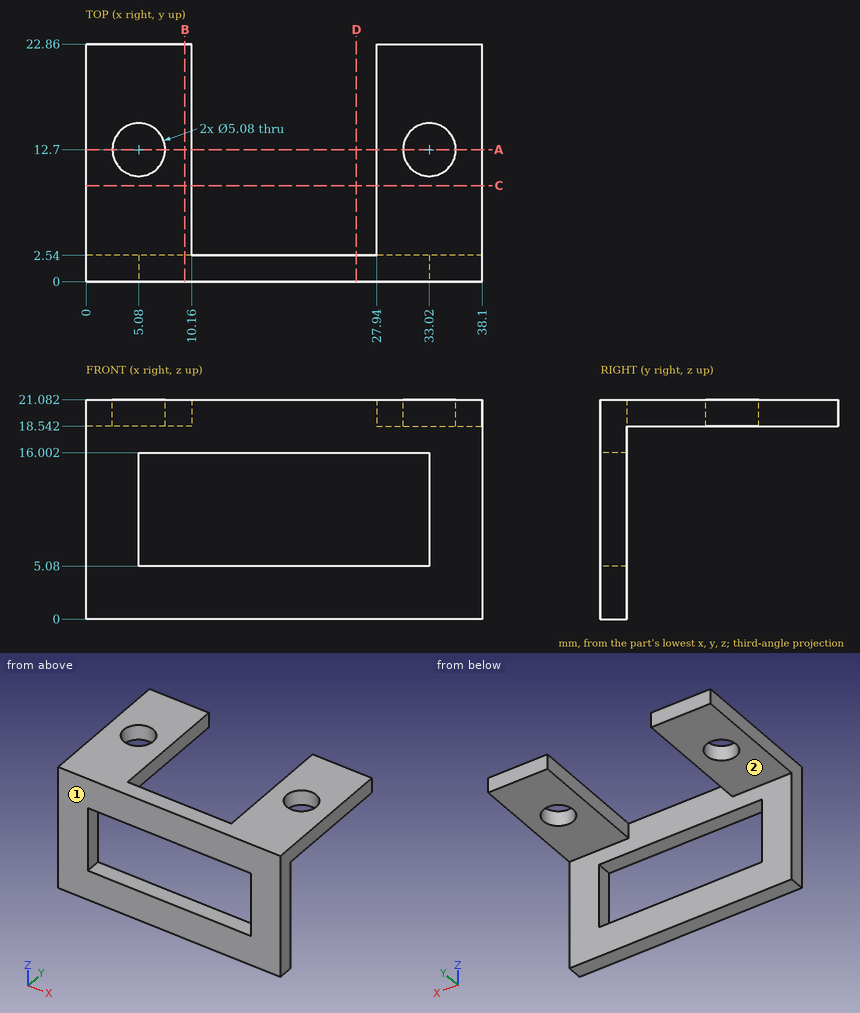
The figure shows three views and two pictorial views of one solid part (mm, origin at its lowest corner). Answer the questions. A direction names the side the tool comes from. Give positions to 0.01 mm unless a question says otherwise; leave off trailing zeros. Loops run counter-clockwise (first coordinate to the right, second up) from the corner with the lowest first, then second, coordinate; pieces in that order, holes last. Notation, with made-up numbers: (25.5, 79) - (57.5, 79) arc R32 ccw to (57.5, 111) - close; hole circle Ø10 at (39, 3.5). An arc over 180 degrees is marked (long way). Use one line per item in the form item = value.
1. Section B-B on x = 9.5 is taken. Give the vertices of the cut face in (y, z), then the cut area to 3 significant figures.
Calculated:
outline = (0, 0) - (2.54, 0) - (2.54, 5.08) - (0, 5.08) - close; (0, 16) - (2.54, 16) - (2.54, 18.54) - (22.86, 18.54) - (22.86, 21.08) - (0, 21.08) - close
area = 77.4 mm^2
2. Section C-C on y = 9.25 is taken. Give the vertices of the cut face in (x, z).
Calculated:
outline = (0, 18.54) - (10.16, 18.54) - (10.16, 21.08) - (0, 21.08) - close; (27.94, 18.54) - (38.1, 18.54) - (38.1, 21.08) - (27.94, 21.08) - close
3. Find the intervals of material crossed by line 1 along X through (y, z) = (12.7, 19.45); line 2 along Y through (x, z) = (33.02, 20); line 3 along Y through (x, z) = (32, 16.75), in increasing order. Write a range as [from, to].
Calculated:
line_1 = [0, 2.54], [7.62, 10.16], [27.94, 30.48], [35.56, 38.1]
line_2 = [0, 10.16], [15.24, 22.86]
line_3 = [0, 2.54]
4. Which of the six approach directions +Z, -Z, +X, -X, +Y, -Y give full straight-line access (tool end or side, diameter ignored) to the marked faces 1 and 2?
Calculated:
face_1 = +Z, -Z, +X, -X, -Y
face_2 = -Z, +X, -X, +Y
5. Section A-A on y = 12.7 is taken. Give the vertices of the cut face in (x, z).
Calculated:
outline = (0, 18.54) - (2.54, 18.54) - (2.54, 21.08) - (0, 21.08) - close; (7.62, 18.54) - (10.16, 18.54) - (10.16, 21.08) - (7.62, 21.08) - close; (27.94, 18.54) - (30.48, 18.54) - (30.48, 21.08) - (27.94, 21.08) - close; (35.56, 18.54) - (38.1, 18.54) - (38.1, 21.08) - (35.56, 21.08) - close
6. Section D-D on x = 26 is taken. Give the vertices of the cut face in (y, z).
Calculated:
outline = (0, 0) - (2.54, 0) - (2.54, 5.08) - (0, 5.08) - close; (0, 16) - (2.54, 16) - (2.54, 21.08) - (0, 21.08) - close
7. Given pin 1 Ø4.5 at (x, y) = (5.08, 12.7) entering from -Z; pin 2 Ø10 at (x, z) = (4.5, 8.5) entering from +Y; pin 3 Ø11 at (x, y) = (4.5, 11.5) entering from -Z, each flat-ended and moving along its own axis, determine where each tip first touches the part or whether it passes through.
Calculated:
pin_1 = through
pin_2 = 2.54
pin_3 = 18.54
